Build history of the part. All positions in model axes, mm. A direction names the side the tool comes from. Round coordinates to 2 decimals unless told otherwise and drop trailing zeros. Loops run counter-clockwise (first coordinate to the right, second up) from the corner with the lowest first, then second, coordinate; pieces in that order, holes last.
from build123d import *

# Parameters (mm, degrees)
PAD003_DEPTH    = 10
SKETCH021_R     = 2.75
PAD009_DEPTH    = 65
SKETCH022_R     = 1.385036
POCKET011_DEPTH = 9
SKETCH043_W     = 2.1
SKETCH043_H     = 1
POCKET021_DEPTH = 0.48
FILLET007_R     = 1


with BuildPart() as part:
    # Sketch007 → Pad003 (new body)
    with BuildSketch(Plane(origin=(-20, 60, -6), x_dir=(1, 0, 0), z_dir=(0, -1, 0))):
        with BuildLine():
            ThreePointArc((44.81, 1.629576), (43.81, 6.941314), (42.81, 1.629576))
            Line((42.81, -1.470424), (42.81, 1.629576))
            Line((44.81, -1.470424), (42.81, -1.470424))
            Line((44.81, 1.629576), (44.81, -1.470424))
        make_face()
    extrude(amount=PAD003_DEPTH)

    # Sketch021 (on Face6 of Pad003) → Pad009 (join)
    with BuildSketch(Plane.XZ.offset(-50)):
        with Locations((23.824507, -1.786051)):
            Circle(SKETCH021_R)
    extrude(amount=PAD009_DEPTH)

    # Sketch022 → Pocket011 (cut)
    with BuildSketch(Plane.XY.offset(2)):
        with Locations((27.12612, -11.774689)):
            Circle(SKETCH022_R)
    extrude(amount=-POCKET011_DEPTH, mode=Mode.SUBTRACT)

    # Sketch043 (on Face7 of Pocket011) → Pocket021 (cut)
    with BuildSketch(Plane(origin=(0, 0, -7.470424), x_dir=(1, 0, 0), z_dir=(0, 0, -1))):
        with Locations((23.804798, -57.3)):
            Rectangle(SKETCH043_W, SKETCH043_H)
        with Locations((23.804798, -52.9)):
            Rectangle(SKETCH043_W, SKETCH043_H)
        with Locations((23.804798, -55.1)):
            Rectangle(SKETCH043_W, SKETCH043_H)
    extrude(amount=-POCKET021_DEPTH, mode=Mode.SUBTRACT)

    # Fillet007
    fillet007_edges = [part.edges().sort_by_distance(p)[0] for p in [
        (23.81, 50, -7.470424),
        (23.81, 60, -7.470424),
    ]]
    fillet(fillet007_edges, radius=FILLET007_R)


with BuildPart() as part_1:
    # Body002 placement: moved
    add(part.part.moved(Location((0, -0.4, -1.5))))


solid = part_1.part
(1) Pin check, flat tips, straight feed: P1, Ø1, axis at y = 7.5, z = -2.5, coming from the -X side; P2, Ø0.5, axis at x = 23.5, z = -8.5, coming from the -Y side; P3, Ø0.9, axis at y = 55.5, z = -7, coming from the +X side; P4, Ø1.5, axis at x = 26, z = -7.5, coming from the -Y side. Stop position of each tip, or through.
Responses:
P1: stops at x = 21.09
P2: stops at y = 49.64
P3: stops at x = 24.81
P4: passes through
(2) Which spindle directions (+Z, -Z, +X, -X, +Y, -Y) get a long thin tool onto all of the face, cutting with end or side? Do faces 1 (the face through (24, -15.4, -3)), 2 (the face through (21.077, 17.555, -3.165)), 3 (the face through (24.81, 55, -7)), 4 (the face through (22.81, 55, -7)), 5 (the face through (24, 58, -8.97)). Say none if no direction does.
Responses:
face 1: +Z, -Z, +X, -X, -Y
face 2: -Y
face 3: -Z, +X, +Y, -Y
face 4: -Z, -X, +Y, -Y
face 5: -Z, +X, -X, +Y, -Y
(3) Probe line 1 (Y direction, x = 25.95, z = -4.75); line 2 (Y direction, x = 25.9, z = -3.5); line 3 (Z direction, x = 23.75, y = 17.5). List the from-to ranges inside material, lowest first.
Responses:
line 1: y = -15.4 to -12.91, -11.44 to 59.6
line 2: y = -15.4 to -12.82, -11.53 to 59.6
line 3: z = -6.04 to -0.54
(4) Slice it at C-C on y = 0. List the corners of the cut face in (x, z), plus the area to 3 significant figures.
Responses:
outline: circle Ø5.5 at (23.82, -3.29)
area: 23.8 mm2
(5) Pull direction Y, two halves, no side cores. Call faces 6 (the face through (25.74, -12.15, -3.26)), 7 (the face through (23.92, 54.67, -0.56)), 8 (the face through (24, 59.6, -3)): +Y half, -Y half, draft (parallel to the pull), parting line (faces both ways), or undercut.
Responses:
face 6: undercut
face 7: draft
face 8: +Y half
